```python
from build123d import *

# Parameters (mm, degrees)
SKETCH_1_W          = 60
SKETCH_1_H          = 65
EXTRUDE_1_DEPTH     = 6
SKETCH_4_R          = 1.5
CUT_EXTRUDE_1_DEPTH = 8
CUT_EXTRUDE_2_DEPTH = 8
SKETCH_7_R          = 1.5
CUT_EXTRUDE_3_DEPTH = 8
SKETCH_8_R          = 1.5
CUT_EXTRUDE_4_DEPTH = 10
FILLET_1_R          = 2


with BuildPart() as part:
    # 草图1 → 凸台-拉伸1 (new body)
    with BuildSketch(Plane(origin=(0, 0, 0), x_dir=(1, 0, 0), z_dir=(0, 1, 0))):
        Rectangle(SKETCH_1_W, SKETCH_1_H)
    extrude(amount=EXTRUDE_1_DEPTH)

    # 草图4 → 切除-拉伸1 (cut)
    with BuildSketch(Plane(origin=(0, 6, 0), x_dir=(1, 0, 0), z_dir=(0, 1, 0))):
        with Locations(Location((-19.60951637, -0.101604527, 0), (0, 0, 270))):
            Circle(SKETCH_4_R)
        with Locations(Location((8.674754878, 28.18266672, 0), (0, 0, 270))):
            Circle(SKETCH_4_R)
        with Locations(Location((-2.638953621, -17.072167276, 0), (0, 0, 270))):
            Circle(SKETCH_4_R)
        with Locations(Location((25.645317626, 11.212103971, 0), (0, 0, 270))):
            Circle(SKETCH_4_R)
    extrude(amount=-CUT_EXTRUDE_1_DEPTH, mode=Mode.SUBTRACT)

    # 草图5 → 切除-拉伸2 (cut)
    with BuildSketch(Plane(origin=(0, 6, 0), x_dir=(1, 0, 0), z_dir=(0, 1, 0))):
        Polygon((-10.140132024, 18.713282374), (-8.189895494, 4.450031542), (-5.526194118, 7.113732918), (-6.63263276, 15.205783111), (1.459417432, 14.099344468), (4.123118808, 16.763045844), align=None)
        Polygon((11.19418662, 9.691978032), (-3.069064212, 11.642214563), (-1.118827682, -2.621036269), (1.544873694, 0.042665106), (0.438435051, 8.134715299), (8.530485244, 7.028276656), align=None)
        Polygon((18.265254432, 2.62091022), (4.0020036, 4.571146751), (5.95224013, -9.692104081), (8.615941506, -7.028402705), (7.509502863, 1.063647487), (15.601553056, -0.042791156), align=None)
    extrude(amount=-CUT_EXTRUDE_2_DEPTH, mode=Mode.SUBTRACT)

    # 草图7 → 切除-拉伸3 (cut)
    with BuildSketch(Plane(origin=(0, 6, 0), x_dir=(1, 0, 0), z_dir=(0, 1, 0))):
        with Locations(Location((-21, -24.5, 0), (0, 0, 270))):
            Circle(SKETCH_7_R)
        with Locations(Location((-21, -16.5, 0), (0, 0, 270))):
            Circle(SKETCH_7_R)
        with Locations(Location((-21, 24.5, 0), (0, 0, 270))):
            Circle(SKETCH_7_R)
        with Locations(Location((-21, 16.5, 0), (0, 0, 270))):
            Circle(SKETCH_7_R)
    extrude(amount=-CUT_EXTRUDE_3_DEPTH, mode=Mode.SUBTRACT)

    # 草图8 → 切除-拉伸4 (cut)
    with BuildSketch(Plane(origin=(0, 6, 0), x_dir=(1, 0, 0), z_dir=(0, 1, 0))):
        Polygon((30, 32.5), (11.42848941, 32.5), (28.399052158, 15.529437252), (24.532691742, -15.959541392), (-6.956286901, -19.825901808), (-23.92684965, -2.855339059), (-23.92684965, 6.144660941), (2.42848941, 32.5), (-30, 32.5), (-30, -32.5), (30, -32.5), align=None)
        with Locations((-21, -24.5)):
            Circle(SKETCH_8_R, mode=Mode.SUBTRACT)
        with Locations((-21, -16.5)):
            Circle(SKETCH_8_R, mode=Mode.SUBTRACT)
        with Locations((-21, 16.5)):
            Circle(SKETCH_8_R, mode=Mode.SUBTRACT)
        with Locations((-21, 24.5)):
            Circle(SKETCH_8_R, mode=Mode.SUBTRACT)
    extrude(amount=-CUT_EXTRUDE_4_DEPTH, mode=Mode.SUBTRACT)

    # 圆角1
    fillet_1_edges = [part.edges().sort_by_distance(p)[0] for p in [
        (2.42848941, 3, -32.5),
        (-23.92684965, 3, -6.144660941),
        (-23.92684965, 3, 2.855339059),
        (-6.956286901, 3, 19.825901808),
        (24.532691742, 3, 15.959541392),
        (28.399052158, 3, -15.529437252),
        (11.42848941, 3, -32.5),
    ]]
    fillet(fillet_1_edges, radius=FILLET_1_R)


solid = part.part
```
Check sheet for the modelled part. Datum: model origin and axes. Units: mm. A direction names the side the tool comes from. Coordinates: 2 decimals unless noted, no trailing zeros. Loops run counter-clockwise (first coordinate to the right, second up) from the corner with the lowest first, then second, coordinate; pieces in that order, holes last.
1) Sectioned sample at A-A (x = 14). Record the boundary of the cut face in (y, z), and give its area (3 significant figures).
2) Gauge pin test, flat ends, axial feed: pin 1 (6 mm diameter, centred on x = -14, z = -1.5, fed in from -Y); pin 2 (1.5 mm diameter, centred on y = 1.5, z = 8.5, fed in from -X); pin 3 (1.5 mm diameter, centred on y = 3.5, z = -1, fed in from +X); pin 4 (1.8 mm diameter, centred on x = 25.65, z = -11.21, fed in from -Y). Record the tip position at first contact, or that the pin passes through.
3) Material ranges on probe 1 along X at (y, z) = (1.75, 0.5); probe 2 along Z at (x, y) = (-1, 3); probe 3 along X at (y, z) = (3, 8), recorded low to high.
4) Sectioned sample at B-B (z = 5). Record the boundary of the cut face in (x, y), and give its area (3 significant figures).
5) Release check for a two-part mould opening along Z. For faces 3 (the face through (26.527, 3.042, -0.279)), 4 (the face through (8.07, 3.04, 3.04)), 5 (the face through (7, 3, -32.5)) record: released by +Z, released by -Z, zero draft, split by the parting line, or undercut.
6) Access from +Z, -Z, +X, -X, +Y, -Y to the whole of each face (thin tool, end or side, straight path). Record for faces 1 (the face through (16.915, 3.042, -1.27)), 2 (the face through (-23.77, 2.96, 2.8)).
7) Sectioned sample at C-C (x = 21.5). Record the boundary of the cut face in (y, z), and give its area (3 significant figures).
8) Sectioned sample at D-D (y = 4.25). Count the separate pieces of the cut face and the enclosed holes in it, and give its area (3 significant figures).
Check sheet entries:
1. outline: (0, -29.93) - (6, -29.93) - (6, -3.2) - (0, -3.2) - close; (0, -0.18) - (6, -0.18) - (6, 17.25) - (0, 17.25) - close
1. area: 265 mm2
2. pin 1: stops at y = 0
2. pin 2: stops at x = -19.03
2. pin 3: stops at x = 26.71
2. pin 4: passes through
3. probe 1: x = -23.93 to -21.06, -18.16 to -1.41, 1 to 4.7, 7.72 to 26.43
3. probe 2: z = -29.07 to -17.46, -14.44 to -11.36, 2.5 to 19.09
3. probe 3: x = -18.78 to 5.72, 7.64 to 25.51
4. outline: (-21.78, 0) - (5.31, 0) - (5.31, 6) - (-21.78, 6) - close; (8.34, 0) - (25.88, 0) - (25.88, 6) - (8.34, 6) - close
4. area: 268 mm2
5. face 3: released by +Z
5. face 4: undercut
5. face 5: released by -Z
6. face 1: +Y, -Y
6. face 2: +Z, -X, +Y, -Y
7. outline: (0, -22.43) - (6, -22.43) - (6, 16.33) - (0, 16.33) - close
7. area: 233 mm2
8. separate pieces: 1
8. enclosed holes: 7
8. area: 1,730 mm2
